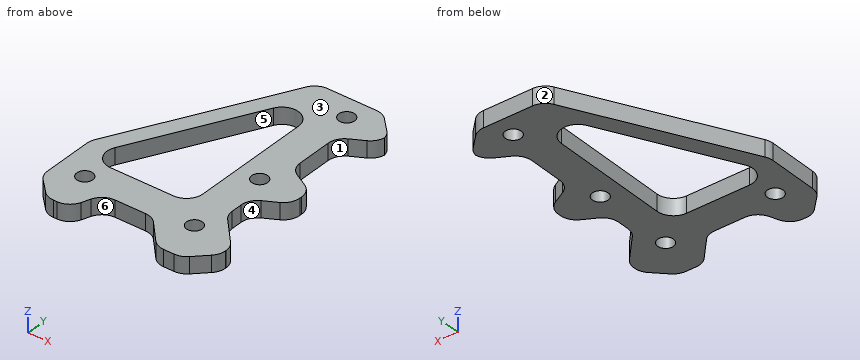
```python
from build123d import *

# Parameters (mm, degrees)
SKETCH_1_R          = 1.45
EXTRUDE_1_DEPTH     = 3
CHAMFER_1_SIZE      = 4
CUT_EXTRUDE_1_DEPTH = 47.421977554
FILLET_1_R          = 3
FILLET_2_R          = 3


with BuildPart() as part:
    # 草图1 → 凸台-拉伸1 (new body)
    with BuildSketch(Plane.XY):
        Polygon((-25, 7.5), (-25, -7.5), (7.5, -7.5), (7.5, 39), (-8.5, 39), align=None)
        with Locations((-20, 0)):
            Circle(SKETCH_1_R, mode=Mode.SUBTRACT)
        Circle(SKETCH_1_R, mode=Mode.SUBTRACT)
        with Locations((0, 15)):
            Circle(SKETCH_1_R, mode=Mode.SUBTRACT)
        with Locations((0, 35)):
            Circle(SKETCH_1_R, mode=Mode.SUBTRACT)
        with BuildLine():
            Line((-9.657494606, 30.324817794), (-21.146102459, 8.392020984))
            ThreePointArc((-21.146102459, 8.392020984), (-21.055323941, 5.446948641), (-18.488607853, 4))
            Line((-18.488607853, 4), (-4, 4))
            Line((-4, 4), (-4, 28.93279681))
            ThreePointArc((-4, 28.93279681), (-6.283230796, 31.845912308), (-9.657494606, 30.324817794))
        make_face(mode=Mode.SUBTRACT)
    extrude(amount=EXTRUDE_1_DEPTH)

    # 倒角1
    chamfer_1_edges = [part.edges().sort_by_distance(p)[0] for p in [
        (7.5, 39, 1.5),
        (7.5, -7.5, 1.5),
        (-25, -7.5, 1.5),
    ]]
    chamfer(chamfer_1_edges, length=CHAMFER_1_SIZE)

    # 草图2 → 切除-拉伸1 (cut, through all)
    with BuildSketch(Plane.XY.offset(3)):
        Polygon((-17, -7.5), (-15, -2), (-6, -2), (-0.958333333, -7.5), align=None)
        Polygon((7.5, 33), (2, 30), (2, 20), (7.5, 17), align=None)
        Polygon((7.5, 13), (2, 10), (2, 5), (7.5, -1), align=None)
    extrude(amount=-CUT_EXTRUDE_1_DEPTH, mode=Mode.SUBTRACT)

    # 圆角1
    fillet_1_edges = [part.edges().sort_by_distance(p)[0] for p in [
        (-4, 4, 1.5),
    ]]
    fillet(fillet_1_edges, radius=FILLET_1_R)

    # 圆角2
    # the kernel refuses this fillet: 3 mm, written as the material it adds along each edge
    with BuildSketch(Plane(origin=(2, 5, 3), x_dir=(0, 1, 0), z_dir=(0, 0, -1))) as fillet_2_piece_1:
        with BuildLine():
            CenterArc((FILLET_2_R * 0.388983690555, FILLET_2_R), FILLET_2_R, 227.489552922, 42.510447078)
            Line((-FILLET_2_R * 0.286740937963, FILLET_2_R * 0.262845859799), (0, 0))
            Line((0, 0), (FILLET_2_R * 0.388983690555, 0))
        make_face()
    extrude(amount=3)
    with BuildSketch(Plane(origin=(2, 10, 3), x_dir=(0.8778955729143842, 0.4788521306805734, 0), z_dir=(0, 0, -1)), Plane(origin=(2, 20, 3), x_dir=(0, 1, 0), z_dir=(0, 0, -1)), Plane(origin=(2, 30, 3), x_dir=(0.8778955729143848, 0.4788521306805725, 0), z_dir=(0, 0, -1))) as fillet_2_piece_2:
        with BuildLine():
            CenterArc((FILLET_2_R * 0.59363309874, FILLET_2_R), FILLET_2_R, 208.610459666, 61.389540334)
            Line((-FILLET_2_R * 0.284262474174, FILLET_2_R * 0.521147869319), (0, 0))
            Line((0, 0), (FILLET_2_R * 0.59363309874, 0))
        make_face()
    extrude(amount=3)
    with BuildSketch(Plane(origin=(-15, -2, 3), x_dir=(1, 0, 0), z_dir=(0, 0, -1))) as fillet_2_piece_3:
        with BuildLine():
            CenterArc((FILLET_2_R * 0.700427264611, FILLET_2_R), FILLET_2_R, 199.983106522, 70.016893478)
            Line((-FILLET_2_R * 0.239366158878, FILLET_2_R * 0.658256936913), (0, 0))
            Line((0, 0), (FILLET_2_R * 0.700427264611, 0))
        make_face()
    extrude(amount=3)
    with BuildSketch(Plane(origin=(-6, -2, 3), x_dir=(0.6757246285173465, -0.7371541402007414, 0), z_dir=(0, 0, -1))) as fillet_2_piece_4:
        with BuildLine():
            CenterArc((FILLET_2_R * 0.439901716342, FILLET_2_R), FILLET_2_R, 222.510447078, 47.489552922)
            Line((-FILLET_2_R * 0.297252423859, FILLET_2_R * 0.324275371483), (0, 0))
            Line((0, 0), (FILLET_2_R * 0.439901716342, 0))
        make_face()
    extrude(amount=3)
    # the kernel refuses this fillet: 3 mm, written as the material it takes off along each edge
    with BuildSketch(Plane(origin=(7.5, 13, 7.452248241), x_dir=(0, 1, 0), z_dir=(0, 0, -1)), Plane(origin=(7.5, 33, 7.452248241), x_dir=(0, 1, 0), z_dir=(0, 0, -1)), Plane(origin=(7.5, 17, 7.452248241), x_dir=(-0.8778955729143842, 0.4788521306805734, 0), z_dir=(0, 0, -1))) as fillet_2_2_piece_1:
        with BuildLine():
            CenterArc((FILLET_2_R * 0.59363309874, -FILLET_2_R), FILLET_2_R, 90, 61.389540334)
            Line((-FILLET_2_R * 0.284262474174, -FILLET_2_R * 0.521147869319), (0, 0))
            Line((0, 0), (FILLET_2_R * 0.59363309874, 0))
        make_face()
    extrude(amount=11.904496481, mode=Mode.SUBTRACT)
    with BuildSketch(Plane(origin=(7.5, -1, 5.917377679), x_dir=(-0.6757246285173458, 0.7371541402007418, 0), z_dir=(0, 0, -1))) as fillet_2_2_piece_2:
        with BuildLine():
            CenterArc((FILLET_2_R * 0.388983690555, -FILLET_2_R), FILLET_2_R, 90, 42.510447078)
            Line((-FILLET_2_R * 0.286740937963, -FILLET_2_R * 0.262845859799), (0, 0))
            Line((0, 0), (FILLET_2_R * 0.388983690555, 0))
        make_face()
    extrude(amount=8.834755358, mode=Mode.SUBTRACT)
    with BuildSketch(Plane(origin=(3.5, -7.5, -3.106601718), x_dir=(0.7071067811865475, 0.7071067811865475, 0), z_dir=(0, 0, 1)), Plane(origin=(-21, -7.5, -3.106601718), x_dir=(1, 0, 0), z_dir=(0, 0, 1)), Plane(origin=(7.5, 35, -3.106601718), x_dir=(-0.7071067811865482, 0.7071067811865468, 0), z_dir=(0, 0, 1)), Plane(origin=(7.5, -3.5, -3.106601718), x_dir=(0, 1, 0), z_dir=(0, 0, 1)), Plane(origin=(3.5, 39, -3.106601718), x_dir=(-1, 0, 0), z_dir=(0, 0, 1))) as fillet_2_2_piece_3:
        with BuildLine():
            CenterArc((FILLET_2_R * 0.414213562373, FILLET_2_R), FILLET_2_R, 225, 45)
            Line((-FILLET_2_R * 0.292893218813, FILLET_2_R * 0.292893218813), (0, 0))
            Line((0, 0), (FILLET_2_R * 0.414213562373, 0))
        make_face()
    extrude(amount=9.213203436, mode=Mode.SUBTRACT)
    with BuildSketch(Plane(origin=(-25, -3.5, -3.106601718), x_dir=(0, 1, 0), z_dir=(0, 0, 1))) as fillet_2_2_piece_4:
        with BuildLine():
            CenterArc((FILLET_2_R * 0.414213562373, -FILLET_2_R), FILLET_2_R, 90, 45)
            Line((-FILLET_2_R * 0.292893218813, -FILLET_2_R * 0.292893218813), (0, 0))
            Line((0, 0), (FILLET_2_R * 0.414213562373, 0))
        make_face()
    extrude(amount=9.213203436, mode=Mode.SUBTRACT)
    with BuildSketch(Plane(origin=(-0.958333333, -7.5, 6.299262873), x_dir=(1, 0, 0), z_dir=(0, 0, -1))) as fillet_2_2_piece_5:
        with BuildLine():
            CenterArc((FILLET_2_R * 0.439901716342, -FILLET_2_R), FILLET_2_R, 90, 47.489552922)
            Line((-FILLET_2_R * 0.297252423859, -FILLET_2_R * 0.324275371483), (0, 0))
            Line((0, 0), (FILLET_2_R * 0.439901716342, 0))
        make_face()
    extrude(amount=9.598525745, mode=Mode.SUBTRACT)
    with BuildSketch(Plane(origin=(-17, -7.5, 8.253204485), x_dir=(0.341743063086704, 0.9397934234884372, 0), z_dir=(0, 0, -1))) as fillet_2_2_piece_6:
        with BuildLine():
            CenterArc((FILLET_2_R * 0.700427264611, -FILLET_2_R), FILLET_2_R, 90, 70.016893478)
            Line((-FILLET_2_R * 0.239366158878, -FILLET_2_R * 0.658256936913), (0, 0))
            Line((0, 0), (FILLET_2_R * 0.700427264611, 0))
        make_face()
    extrude(amount=13.506408969, mode=Mode.SUBTRACT)
    with BuildSketch(Plane(origin=(-8.5, 39, -4.538049708), x_dir=(-0.464006994670558, -0.8858315352801552, 0), z_dir=(0, 0, 1))) as fillet_2_2_piece_7:
        with BuildLine():
            CenterArc((FILLET_2_R * 0.605073294393, FILLET_2_R), FILLET_2_R, 207.645975364, 62.354024636)
            Line((-FILLET_2_R * 0.280758240887, FILLET_2_R * 0.535993005329), (0, 0))
            Line((0, 0), (FILLET_2_R * 0.605073294393, 0))
        make_face()
    extrude(amount=12.076099416, mode=Mode.SUBTRACT)
    with BuildSketch(Plane(origin=(-25, 7.5, -1.845367624), x_dir=(0, -1, 0), z_dir=(0, 0, 1))) as fillet_2_2_piece_8:
        with BuildLine():
            CenterArc((FILLET_2_R * 0.246049016569, FILLET_2_R), FILLET_2_R, 242.354024636, 27.645975364)
            Line((-FILLET_2_R * 0.217957978102, FILLET_2_R * 0.11416846472), (0, 0))
            Line((0, 0), (FILLET_2_R * 0.246049016569, 0))
        make_face()
    extrude(amount=6.690735249, mode=Mode.SUBTRACT)


solid = part.part
```
Design review of the part built by this model. Coordinates are the model's own, in mm. Face numbers are marked on the shaded views. A direction names the side the tool comes from. Coordinates: 2 decimals unless noted, no trailing zeros. Loops run counter-clockwise (first coordinate to the right, second up) from the corner with the lowest first, then second, coordinate; pieces in that order, holes last.
Q1. We need section B-B on y = 35. State the section outline as (x, z) points, and give its area (3 significant figures).
Reported:
outline: (-10.6, 0) - (-1.45, 0) - (-1.45, 3) - (-10.6, 3) - close; (1.45, 0) - (7.23, 0) - (7.23, 3) - (1.45, 3) - close
area: 44.8 mm2
Q2. To check wall thickness, follow line 1 (X direction, y = 0.5, z = 2.7) (3 decimals); line 2 (Y direction, x = -20, z = 0.2); line 3 (Y direction, x = -21, z = 2.6). State the ranges of each line that lie inside material, in increasing order.
Reported:
line 1: x = -25 to -21.361, -18.639 to -1.361, 1.361 to 6.125
line 2: y = -7.49 to -1.45, 1.45 to 4.41, 10.58 to 17.05
line 3: y = -7.23 to -1.05, 1.05 to 5.36, 8.67 to 15.14
Q3. The part is to be moulded in two halves that separate along Y. For the marked faces 1, 2 and 3, say which applies: +Y half, -Y half, draft (parallel to the pull), parting line (faces both ways), or undercut.
Reported:
face 1: undercut
face 2: +Y half
face 3: draft
Q4. For pin 1 (1.5 mm diameter, centred on y = 24, z = 1.5, fed in from +X); pin 2 (0.9 mm diameter, centred on y = 15, z = 2, fed in from -X); pin 3 (1.5 mm diameter, centred on x = -10.5, z = 1.5, fed in from -Y); pin 4 (1.7 mm diameter, centred on x = 0, y = 15, fed in from -Z), all flat-tipped, find the tip position at first contact; note any pin that passes through.
Reported:
pin 1: stops at x = 2
pin 2: stops at x = -21.31
pin 3: stops at y = -2
pin 4: passes through
Q5. We need section A-A on x = -8.5. State the section outline as (y, z) points, and give its area (3 significant figures).
Reported:
outline: (-2, 0) - (4, 0) - (4, 3) - (-2, 3) - close; (31.53, 0) - (38.39, 0) - (38.39, 3) - (31.53, 3) - close
area: 38.6 mm2
Q6. We need section C-C on z = 0.5. State how many separate pieces and enclosed holes the cut face has, and give its area (3 significant figures).
Reported:
separate pieces: 1
enclosed holes: 5
area: 678 mm2
Q7. Tool access review of the marked faces 4, 5 and 6: name each direction out of +Z, -Z, +X, -X, +Y, -Y from which nothing blocks a thin tool from reaching the whole face with its end or side.
Reported:
face 4: +Z, -Z, +X
face 5: +Z, -Z
face 6: +Z, -Z, -Y
